The listing builds one solid part. Answer for the finished solid, in the listing's coordinates (mm). A direction names the side the tool comes from. Coordinates: 2 decimals unless noted, no trailing zeros. Order: outer loops, then holes, each group sorted by start corner. A loop starts at its lowest first (then second) coordinate and runs counter-clockwise, first axis right, second up. Notation, with made-up numbers: (82.5, 76) -> (119.5, 76) arc R22 ccw to (119.5, 88) -> close; hole circle Ø6 at (0, 87). An arc over 180 degrees is marked (long way). Write item = value, one per line. Start each with the question number.
Autodesk Fusion 360 part; units mm, degrees
sketch "Sketch1" plane through (0, 0, 0) normal (0, 0, 1) x (1, 0, 0)
  line L0 (-40, 50) -> (210, 50)
  line L1 (210, 50) -> (210, -100)
  line L2 (210, -100) -> (-40, -100)
  line L3 (-40, -100) -> (-40, 50)
  line L4 (-35, 45) -> (205, 45)
  line L5 (205, 45) -> (205, -95)
  line L6 (205, -95) -> (-35, -95)
  line L7 (-35, -95) -> (-35, 45)
  dimension "d1" = 250
  dimension "d2" = 150
  dimension "d3" = 5
  dimension "d4" = 5
  dimension "d5" = 5
  dimension "d6" = 5
sketch "Sketch2" plane through (0, 0, 0) normal (0, 0, 1) x (1, 0, 0)
  circle A0 centre (185, 15) radius 3.5
  line L0 (205, 45) -> (205, -95)
  line L1 (-35, 45) -> (205, 45)
  dimension "d7" = 7
  dimension "d8" = 20
  dimension "d9" = 30
  dimension "d12" = 20
sketch "Sketch3" plane through (0, 0, 0) normal (0, 0, 1) x (1, 0, 0)
extrude "Extrude1" add sketch "Sketch1" along normal blind 100
sketch "Sketch4" plane through (0, 0, 0) normal (0, 1, 0) x (1, 0, 0)
sketch "Sketch5" plane through (0, 0, 0) normal (0, 0, 1) x (1, 0, 0)
  line L0 (-35, 45) -> (205, 45)
  line L1 (205, 45) -> (205, -95)
  line L2 (205, -95) -> (-35, -95)
  line L3 (-35, -95) -> (-35, 45)
extrude "Extrude2" add sketch "Sketch5" along normal blind 10
sketch "Sketch6" plane through (0, 0, 10) normal (0, 0, 1) x (-1, 0, 0)
  line L0 (35, 95) -> (-205, 95)
  line L1 (-205, 95) -> (-205, -45)
  line L2 (-205, -45) -> (35, -45)
  line L3 (35, -45) -> (35, 95)
  circle A0 centre (-185, -15) radius 3.6056
extrude "Extrude3" cut sketch "Sketch6" against normal blind 10 contours A0
sketch "Sketch7" plane through (0, 0, 0) normal (0, 0, 1) x (1, 0, 0)
  line L0 (-20, -50) -> (5.5, -50)
  line L1 (5.5, -50) -> (5.5, -35.9)
  line L2 (5.5, -35.9) -> (-20, -35.9)
  line L3 (-20, -35.9) -> (-20, -50)
  line L4 (210, -100) -> (-40, -100)
  dimension "d20" = 25.5
  dimension "d21" = 14.1
  dimension "d22" = 50
extrude "Extrude4" cut sketch "Sketch7" along normal blind 10
sketch "Sketch8" plane through (0, 0, 10) normal (0, 0, 1) x (-1, 0, 0)
  line L0 (20, 35.9) -> (-5.5, 35.9)
  line L1 (-5.5, 35.9) -> (-5.5, 50)
  line L2 (-5.5, 50) -> (20, 50)
  line L3 (20, 50) -> (20, 35.9)
  circle A0 centre (-185, -15) radius 3.6056
  line L4 (35, 95) -> (-205, 95)
  line L5 (-205, 95) -> (-205, -45)
  line L6 (-205, -45) -> (35, -45)
  line L7 (35, -45) -> (35, 95)
  line L8 (22.8, 30.9) -> (-7.2, 30.9)
  line L9 (-7.2, 30.9) -> (-7.2, 59.9)
  line L10 (-7.2, 59.9) -> (22.8, 59.9)
  line L11 (22.8, 59.9) -> (22.8, 30.9)
  dimension "d25" = 30
  dimension "d26" = 29
  dimension "d27" = 5
  dimension "d28" = 1.7
  dimension "d29" = 29
extrude "Extrude5" cut sketch "Sketch8" against normal blind 7 contours L8 L9 L10 L11
sketch "Sketch9" plane through (0, 0, 10) normal (0, 0, 1) x (-1, 0, 0)
  line L0 (-7.2, 30.9) -> (-7.2, 59.9)
  line L1 (-7.2, 59.9) -> (22.8, 59.9)
  line L2 (22.8, 59.9) -> (22.8, 30.9)
  line L3 (22.8, 30.9) -> (-7.2, 30.9)
  circle A0 centre (-185, -15) radius 3.6056
  line L4 (35, 95) -> (-205, 95)
  line L5 (-205, 95) -> (-205, -45)
  line L6 (-205, -45) -> (35, -45)
  line L7 (35, -45) -> (35, 95)
sketch "Sketch10" plane through (0, 0, 10) normal (0, 0, 1) x (-1, 0, 0)
sketch "Sketch11" plane through (0, 0, 10) normal (0, 0, 1) x (-1, 0, 0)
  line L0 (34.9, -32.7882) -> (-25.2, -32.7882)
  line L1 (-25.2, -32.7882) -> (-25.2, 17.7118)
  line L2 (-25.2, 17.7118) -> (34.9, 17.7118)
  line L3 (34.9, 17.7118) -> (34.9, -32.7882)
  line L4 (35.6, -7.5382) -> (29.9, -7.5382)
  line L5 (29.9, -7.5382) -> (29.9, -15.5382)
  line L6 (29.9, -15.5382) -> (35.6, -15.5382)
  line L7 (35.6, -15.5382) -> (35.6, -7.5382)
  line L8 (35, 95) -> (35, -45)
  dimension "d38" = 60.1
  dimension "d39" = 50.5
  dimension "d40" = 5.7
  dimension "d41" = 8
  dimension "d42" = 55.1
  dimension "d43" = 0.1
sketch "Sketch12" plane through (0, 0, 0) normal (1, 0, 0) x (0, 1, 0)
sketch "Sketch13" plane through (-40, 0, 0) normal (-1, 0, 0) x (0, -1, 0)
  line L0 (-50, 0) -> (100, 0)
  line L1 (100, 0) -> (100, 100)
  line L2 (100, 100) -> (-50, 100)
  line L3 (-50, 100) -> (-50, 0)
  line L4 (-19.2882, 18) -> (-4.2882, 18)
  line L5 (-4.2882, 18) -> (-4.2882, 3)
  line L6 (-4.2882, 3) -> (-19.2882, 3)
  line L7 (-19.2882, 3) -> (-19.2882, 18)
  line L8 (-15.5382, 10) -> (-7.5382, 10)
  dimension "d44" = 15
  dimension "d45" = 15
  dimension "d46" = 8
  dimension "d47" = 3.75
extrude "Extrude6" cut sketch "Sketch13" against normal blind 13 contours L4 L5 L6 L7
extrude "Extrude7" cut sketch "Sketch11" against normal blind 3 contours L0 L1 L2 L3 L4 L5 L6
sketch "Sketch14" plane through (0, 0, 0) normal (0, 0, 1) x (1, 0, 0)
sketch "Sketch15" plane through (0, 0, 0) normal (0, 0, 1) x (1, 0, 0)
sketch "Sketch16" plane through (0, -100, 0) normal (0, -1, 0) x (1, 0, 0)
  line L0 (-40, 0) -> (210, 0)
  line L1 (210, 0) -> (210, 100)
  line L2 (210, 100) -> (-40, 100)
  line L3 (-40, 100) -> (-40, 0)
  line L4 (10, 40) -> (20.2, 40)
  line L5 (20.2, 40) -> (20.2, 30)
  line L6 (20.2, 30) -> (10, 30)
  line L7 (10, 30) -> (10, 40)
  line L8 (205, 0) -> (-35, 0)
  dimension "d52" = 10.2
  dimension "d53" = 10
  dimension "d54" = 30
  dimension "d55" = 50
extrude "Extrude8" cut sketch "Sketch16" against normal blind 10 contours L4 L5 L6 L7
sketch "Sketch17" plane through (-40, 0, 0) normal (-1, 0, 0) x (0, -1, 0)
  line L0 (-4.2882, 18) -> (-4.2882, 3)
  line L1 (-4.2882, 3) -> (-19.2882, 3)
  line L2 (-19.2882, 3) -> (-19.2882, 18)
  line L3 (-19.2882, 18) -> (-4.2882, 18)
  line L4 (-50, 0) -> (100, 0)
  line L5 (100, 0) -> (100, 100)
  line L6 (100, 100) -> (-50, 100)
  line L7 (-50, 100) -> (-50, 0)
  line L8 (-19.2882, 18) -> (-4.2882, 18)
  line L9 (-4.2882, 18) -> (-4.2882, 3)
  line L10 (-4.2882, 3) -> (-19.2882, 3)
  line L11 (-19.2882, 3) -> (-19.2882, 18)
extrude "Extrude9" add sketch "Sketch17" against normal blind 13 contours L0 L1 L2 L3 L8 L9 L10 L11
sketch "Sketch18" plane through (0, 0, 10) normal (0, 0, 1) x (-1, 0, 0)
  line L0 (26.9999, 2.0114) -> (35, 2.0114)
  line L1 (35, 2.0114) -> (35, -15.984)
  line L2 (35, -15.984) -> (26.9999, -15.984)
  line L3 (26.9999, -15.984) -> (26.9999, 2.0114)
extrude "Extrude10" cut 1 faces at (-32.3333, 14.2882, 18) along direction (0, 0, -1) blind 11
extrude "Extrude11" cut sketch "Sketch18" against normal blind 4
sketch "Sketch19" plane through (-35, 0, 0) normal (1, 0, 0) x (0, 1, 0)
  line L0 (15.984, 7) -> (19.2882, 7)
  line L1 (19.2882, 7) -> (19.2882, 10)
  line L2 (19.2882, 10) -> (45, 10)
  line L3 (45, 10) -> (45, 100)
  line L4 (45, 100) -> (-95, 100)
  line L5 (-95, 100) -> (-95, 10)
  line L6 (-95, 10) -> (-2.0114, 10)
  line L7 (-2.0114, 10) -> (-2.0114, 6)
  line L8 (-2.0114, 6) -> (15.984, 6)
  line L9 (15.984, 6) -> (15.984, 7)
  line L10 (-2.0114, 10) -> (15.984, 10)
  line L11 (-2.0114, 7) -> (-2.0114, 10)
sketch "Sketch20" plane through (-35, 0, 0) normal (1, 0, 0) x (0, 1, 0)
sketch "Sketch21" plane through (-35, 0, 0) normal (1, 0, 0) x (0, 1, 0)
  line L0 (-2, 10) -> (16, 10)
  line L1 (16, 10) -> (16, 7)
  line L2 (16, 7) -> (-2, 7)
  line L3 (-2, 7) -> (-2, 10)
sketch "Sketch22" plane through (-40, 0, 0) normal (-1, 0, 0) x (0, -1, 0)
  line L0 (-50, 0) -> (100, 0)
  line L1 (100, 0) -> (100, 100)
  line L2 (100, 100) -> (-50, 100)
  line L3 (-50, 100) -> (-50, 0)
  line L4 (-16, 10) -> (2, 10)
  line L5 (2, 10) -> (2, 7)
  line L6 (2, 7) -> (-16, 7)
  line L7 (-16, 7) -> (-16, 10)
extrude "Extrude12" cut sketch "Sketch22" against normal blind 6 contours L4 L5 L6 L7
sketch "Sketch23" plane through (-35, 0, 0) normal (1, 0, 0) x (0, 1, 0)
sketch "Sketch24" plane through (-40, 0, 0) normal (-1, 0, 0) x (0, -1, 0)
  line L0 (2, 10) -> (2, 7)
  line L1 (2, 7) -> (-16, 7)
  line L2 (-16, 7) -> (-16, 10)
  line L3 (-16, 10) -> (2, 10)
  line L4 (-50, 0) -> (100, 0)
  line L5 (100, 0) -> (100, 100)
  line L6 (100, 100) -> (-50, 100)
  line L7 (-50, 100) -> (-50, 0)
  line L8 (-16, 14) -> (2, 14)
  line L9 (2, 14) -> (2, 6)
  line L10 (2, 6) -> (-16, 6)
  line L11 (-16, 6) -> (-16, 14)
extrude "Extrude13" cut sketch "Sketch24" against normal blind 58 contours L3 L8 L9 L11
sketch "Sketch25" plane through (-35, 0, 0) normal (1, 0, 0) x (0, 1, 0)
extrude "Extrude14" add sketch "Sketch21" against normal blind 5
sketch "Sketch26" plane through (-35, 0, 0) normal (1, 0, 0) x (0, 1, 0)
  line L0 (16, 14) -> (-2, 14)
  line L1 (-2, 14) -> (-2, 10)
  line L2 (-2, 10) -> (16, 10)
  line L3 (16, 10) -> (16, 14)
extrude "Extrude15" add sketch "Sketch26" against normal blind 5
sketch "Sketch27" plane through (0, 0, 10) normal (0, 0, 1) x (-1, 0, 0)
  line L0 (27, 12) -> (35, 12)
  line L1 (35, 12) -> (35, 2)
  line L2 (35, 2) -> (27, 2)
  line L3 (27, 2) -> (27, 12)
extrude "Extrude16" cut sketch "Sketch27" against normal blind 4
sketch "Sketch28" plane through (0, 0, 10) normal (0, 0, 1) x (-1, 0, 0)
sketch "Sketch29" plane through (0, 0, 10) normal (0, 0, 1) x (-1, 0, 0)
sketch "Sketch30" plane through (0, 0, 0) normal (1, 0, 0) x (0, 1, 0)
sketch "Sketch31" plane through (-40, 0, 0) normal (-1, 0, 0) x (0, -1, 0)
  line L0 (-50, 0) -> (100, 0)
  line L1 (100, 0) -> (100, 100)
  line L2 (100, 100) -> (-50, 100)
  line L3 (-50, 100) -> (-50, 0)
  line L4 (-12.7294, 18) -> (11.2444, 18)
  line L5 (11.2444, 18) -> (11.2444, 5)
  line L6 (11.2444, 5) -> (-12.7294, 5)
  line L7 (-12.7294, 5) -> (-12.7294, 18)
extrude "Extrude17" cut sketch "Sketch31" against normal blind 13 contours L4 L5 L6 L7
Item 1: Section B-B, the plane z = 48 is taken. Give the vertices of the cut face in (x, y).
Item 2: Section D-D, the plane x = 16.5 is taken. Give the vertices of the cut face in (y, z), then the cut area to 3 significant figures.
Item 3: Each of these flat-tipped pins is pushed along its axis until it touches: pin 1 (4 mm diameter, centred on x = 36.5, y = -28, fed in from -Z); pin 2 (12 mm diameter, centred on x = 110, y = -33, fed in from +Z); pin 3 (0.5 mm diameter, centred on y = 3, z = 6.5, fed in from -X). Where does it stop, or does it pass through?
Item 4: Which of the six approach directions +Z, -Z, +X, -X, +Y, -Y give full straight-line access (tool end or side, diameter ignored) to faces 4 (the flat face through (20.2, -98, 35)), 5 (the flat face through (-36, 12.729, 11)), 6 (the flat face through (87, -95, 54)), 7 (the cylindrical face through (188.6, 14.8, 5.1))?
Item 5: Consider probe 1 along X at (y, z) = (15, 6.5); probe 2 along X at (y, z) = (-28, 44.5); probe 3 along X at (y, z) = (15, 5.25). Determine where each line is inside the solid, lowest interval first.
Item 6: Section C-C, the plane y = 37.5 is taken. Give the vertices of the cut face in (x, z).
Item 7: Section A-A, the plane x = 185 is taken. Give the vertices of the cut face in (y, z).
Item 8: For a pull along Y with two mould halves and no side action, classify faces 1 (the flat face through (83, 50, 49)), 2 (the flat face through (-34, 1, 5)), 3 (the flat face through (15, -98, 30)) as pulls with the +Y half, pulls with the -Y half, needs draft (parallel to the pull), parting line crosses it, or undercut.
A:
q1.outline = (-40, -100) -> (210, -100) -> (210, 50) -> (-40, 50) -> close; hole (-35, -95) -> (205, -95) -> (205, 45) -> (-35, 45) -> close
q2.outline = (-100, 0) -> (50, 0) -> (50, 100) -> (45, 100) -> (45, 10) -> (32.79, 10) -> (32.79, 7) -> (-17.71, 7) -> (-17.71, 10) -> (-95, 10) -> (-95, 30) -> (-100, 30) -> close; (-100, 40) -> (-95, 40) -> (-95, 100) -> (-100, 100) -> close
q2.area = 2,200 mm^2
q3.pin_1 = 0
q3.pin_2 = 10
q3.pin_3 = -27
q4.face_4 = -Y
q4.face_5 = -X
q4.face_6 = +Z
q4.face_7 = +Z, -Z
q5.probe_1 = -40 to -35, -27 to 181.39, 188.61 to 210
q5.probe_2 = -40 to -35, 205 to 210
q5.probe_3 = -40 to 181.39, 188.61 to 210
q6.outline = (-40, 0) -> (210, 0) -> (210, 100) -> (205, 100) -> (205, 10) -> (-35, 10) -> (-35, 100) -> (-40, 100) -> close
q7.outline = (-100, 0) -> (11.39, 0) -> (11.39, 10) -> (-95, 10) -> (-95, 100) -> (-100, 100) -> close; (18.61, 0) -> (50, 0) -> (50, 100) -> (45, 100) -> (45, 10) -> (18.61, 10) -> close
q8.face_1 = pulls with the +Y half
q8.face_2 = undercut
q8.face_3 = needs draft
